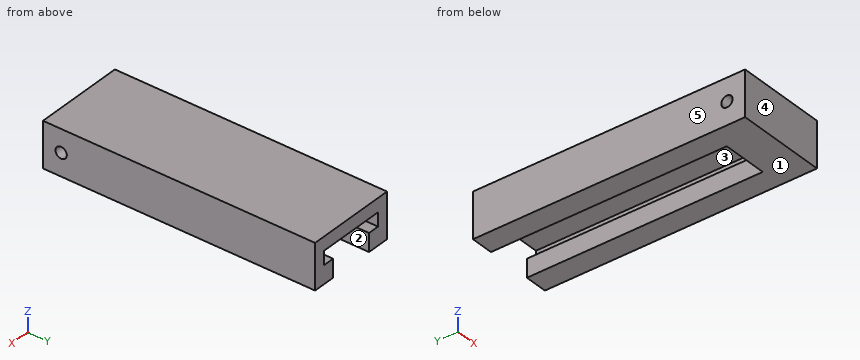
```python
from build123d import *

# Parameters (mm, degrees)
SZKIC1_W                    = 40
SZKIC1_H                    = 20
DODANIE_WYCI_GNI_CIE1_DEPTH = 120
SZKIC2_R                    = 2.5
WYTNIJ_WYCI_GNI_CIE1_DEPTH  = 127.885775404
WYTNIJ_WYCI_GNI_CIE2_DEPTH  = 104


with BuildPart() as part:
    # Szkic1 → Dodanie-wyciągnięcie1 (new body)
    with BuildSketch(Plane(origin=(0, 0, 0), x_dir=(1, 0, 0), z_dir=(0, 1, 0))):
        Rectangle(SZKIC1_W, SZKIC1_H)
    extrude(amount=DODANIE_WYCI_GNI_CIE1_DEPTH)

    # Szkic2 → Wytnij-wyciągnięcie1 (cut, through all)
    with BuildSketch(Plane.ZY.offset(20)):
        with Locations((0, 8)):
            Circle(SZKIC2_R)
    extrude(amount=-WYTNIJ_WYCI_GNI_CIE1_DEPTH, mode=Mode.SUBTRACT)

    # Szkic4 → Wytnij-wyciągnięcie2 (cut)
    with BuildSketch(Plane(origin=(0, 120, 0), x_dir=(1, 0, 0), z_dir=(0, 1, 0))):
        Polygon((-15, -4), (15, -4), (15, 2), (10, 2), (10, 10), (-10, 10), (-10, 2), (-15, 2), align=None)
    extrude(amount=-WYTNIJ_WYCI_GNI_CIE2_DEPTH, mode=Mode.SUBTRACT)


solid = part.part
```
Input: part model. Units: mm. Frame: model coordinates. Face numbers are marked on the shaded views. A direction names the side the tool comes from. Round coordinates to 2 decimals unless told otherwise and drop trailing zeros. Loops run counter-clockwise (first coordinate to the right, second up) from the corner with the lowest first, then second, coordinate; pieces in that order, holes last. Notation, with made-up numbers: M 31,74.25 L 46,74.25 A17 ccw 46,87.25 Z; hole C -21,-39 d8. An arc over 180 degrees is marked long. Answer in a Markdown table with one row per item. Add a question column.
1. Mould query, pull axis X, two halves, no side actions, for the marked faces 3, 4 and 5. Classes: released by +X, released by -X, zero draft, split by the parting line, or undercut.
2. Section B-B (x = -13). Output: boundary loops of the cut face in (y, z).
3. Section D-D (y = 54). Output: boundary loops of the cut face in (x, z), and give its area (3 significant figures).
4. Section A-A (y = 8). Output: boundary loops of the cut face in (x, z).
5. Contact query for a flat-ended pin moving along its axis: pin 1 (7 mm diameter, centred on x = 5.5, z = -4, fed in from +Y). Output: stop coordinate, or through.
6. Ray query, probe 1 along Y at (x, z) = (-9.5, 0); probe 2 along X at (y, z) = (60.5, 2.25); probe 3 along Z at (x, y) = (-10.5, 46). Return the intervals inside material, ascending.
7. Section C-C (z = 0). Output: boundary loops of the cut face in (x, y).
8. Set-up query: the marked faces 1 and 2. Return all of +Z, -Z, +X, -X, +Y, -Y with unobstructed straight access to the full face (end or side cutting, diameter ignored); none if empty.
Values follow:
| question | item | result |
|---|---|---|
| 1 | face 3 | undercut |
| 1 | face 4 | zero draft |
| 1 | face 5 | released by -X |
| 2 | outline | M 0,-10 L 120,-10 L 120,-2 L 16,-2 L 16,4 L 120,4 L 120,10 L 0,10 Z; hole C 8,0 d5 |
| 3 | outline | M -20,-10 L -10,-10 L -10,-2 L -15,-2 L -15,4 L 15,4 L 15,-2 L 10,-2 L 10,-10 L 20,-10 L 20,10 L -20,10 Z |
| 3 | area | 460 mm^2 |
| 4 | outline | M -20,-10 L 20,-10 L 20,-2.5 L -20,-2.5 Z; M -20,2.5 L 20,2.5 L 20,10 L -20,10 Z |
| 5 | pin 1 | y = 16 |
| 6 | probe 1 | 0 to 5.5, 10.5 to 16 |
| 6 | probe 2 | -20 to -15, 15 to 20 |
| 6 | probe 3 | -10 to -2, 4 to 10 |
| 7 | outline | M -20,0 L 20,0 L 20,5.5 L -20,5.5 Z; M -20,10.5 L 20,10.5 L 20,120 L 15,120 L 15,16 L -15,16 L -15,120 L -20,120 Z |
| 8 | face 1 | -Z, +X, -X, +Y, -Y |
| 8 | face 2 | -Z, +Y |
